Geometry: final body of the model. Coordinates: model frame, mm. A direction names the side the tool comes from. Give positions to 0.01 mm unless a question says otherwise; leave off trailing zeros. Write each loop counter-clockwise with the first axis right and the second up, starting at its lowest first coordinate (ties: lowest second). Pieces come first, ordered by that corner, then holes.
Q1. Cut plane B-B on z = 35. Return the cut outline in (x, y).
Q2. Reachability of faces 1 (the face through (-17.305, 0, 34)), 2 (the face through (-52, 0, 15.035)), 3 (the face through (-48.305, 0, 32)), 4 (the face through (-32, 0, 57.035)) from +Z, -Z, +X, -X, +Y, -Y: full face, straight path, thin tool, end or side. Return the list, or none.
Q3. Pin query (flat end, axial travel): pin 1 (7 mm diameter, centred on x = -34, y = 1.5, fed in from -Z); pin 2 (5 mm diameter, centred on x = -36.31, y = 0, fed in from +Z); pin 3 (9 mm diameter, centred on x = -1.5, y = -3.5, fed in from +Z). Return the tip coordinate at first contact, or that it passes through.
Q4. Cut plane A-A on y = 0. Return the cut outline in (x, z).
Q5. Cut plane C-C on y = -10. Return the cut outline in (x, z).
Q6. Cut plane D-D on x = -14. Return the cut outline in (y, z), plus the area to 3 significant figures.
Q7. Line query: L1, parallel to X at y = 0, z = 51.85; L2, parallel to X at y = -2.75, z = 42; L3, parallel to Z at x = -46, y = 6.25. Output: solid intervals per line, ascending.
Q8. Draft query along Y for faces 5 (the face through (-24, -15, 31)), 6 (the face through (-6, 0, 4.035)), 7 (the face through (1.19, 0.15, 7.49)). Return one class per face: pulls with the +Y half, pulls with the -Y half, needs draft (parallel to the pull), parting line crosses it, or undercut.
```python
from build123d import *

# Parameters (mm, degrees)
F1_DEPTH       = 15
F3_D           = 7
F5_D           = 4.5
F5_CSINK_D     = 8
F5_CSINK_ANGLE = 90


with BuildPart() as f1:
    # F0 (on Front) → F1 (new body, symmetric)
    with BuildSketch(Plane.XZ):
        Polygon((-55.305267, 15.034918), (-48.305267, 15.034918), (-48.305267, 50.034918), (-24.305267, 50.034918), (-24.305267, 4.034918), (12.694733, 4.034918), (12.694733, 11.034918), (-17.305267, 11.034918), (-17.305267, 57.034918), (-55.305267, 57.034918), align=None)
    extrude(amount=F1_DEPTH, both=True)

    # F3 (through all)
    with Locations(Plane.XY.offset(11.034918)):
        with Locations((-2.305267, 0)):
            Hole(F3_D / 2)

    # F5 (through all)
    with Locations(Plane.XY.offset(57.034918)):
        with Locations((-36.305267, 0)):
            CounterSinkHole(F5_D / 2, F5_CSINK_D / 2, counter_sink_angle=F5_CSINK_ANGLE)


solid = f1.part
```
Data:
1. outline: (-55.31, -15) - (-48.31, -15) - (-48.31, 15) - (-55.31, 15) - close; (-24.31, -15) - (-17.31, -15) - (-17.31, 15) - (-24.31, 15) - close
2. face 1: +Z, +X, +Y, -Y
2. face 2: -Z, -X, +Y, -Y
2. face 3: -Z, +Y, -Y
2. face 4: +Z, +X, -X, +Y, -Y
3. pin 1: stops at z = 50.03
3. pin 2: stops at z = 55.54
3. pin 3: stops at z = 11.03
4. outline: (-55.31, 15.03) - (-48.31, 15.03) - (-48.31, 50.03) - (-38.56, 50.03) - (-38.56, 55.28) - (-40.31, 57.03) - (-55.31, 57.03) - close; (-34.06, 50.03) - (-24.31, 50.03) - (-24.31, 4.03) - (-5.81, 4.03) - (-5.81, 11.03) - (-17.31, 11.03) - (-17.31, 57.03) - (-32.31, 57.03) - (-34.06, 55.28) - close; (1.19, 4.03) - (12.69, 4.03) - (12.69, 11.03) - (1.19, 11.03) - close
5. outline: (-55.31, 15.03) - (-48.31, 15.03) - (-48.31, 50.03) - (-24.31, 50.03) - (-24.31, 4.03) - (12.69, 4.03) - (12.69, 11.03) - (-17.31, 11.03) - (-17.31, 57.03) - (-55.31, 57.03) - close
6. outline: (-15, 4.03) - (15, 4.03) - (15, 11.03) - (-15, 11.03) - close
6. area: 210 mm2
7. L1: x = -55.31 to -38.56, -34.06 to -17.31
7. L2: x = -55.31 to -48.31, -24.31 to -17.31
7. L3: z = 50.03 to 57.03
8. face 5: pulls with the -Y half
8. face 6: needs draft
8. face 7: undercut
